Answer from the drawing. Dimensions are ordinates in mm from the lowest x, y and z of the part. A direction names the side the tool comes from. Give positions to 0.01 mm unless a question says otherwise; leave off trailing zeros. Loops run counter-clockwise (first coordinate to the right, second up) from the corner with the lowest first, then second, coordinate; pieces in that order, holes last. Notation, with made-up numbers: M 63.5,25 L 100.5,25 A25 cw 100.5,47 Z; hole C 28.25,82 d9. An arc over 180 degrees is marked long. Use a Markdown table: item, result.
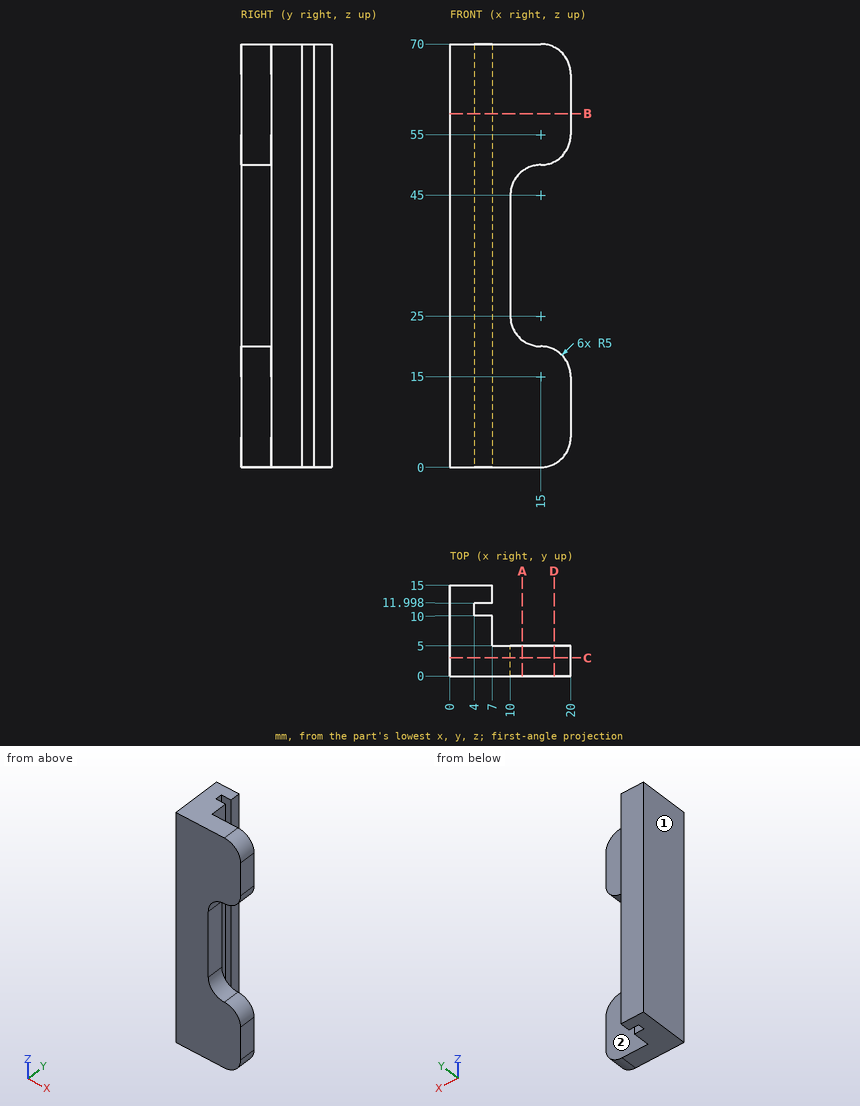
(1) Consider probe 1 along Y at (x, z) = (5, 40); probe 2 along X at (y, z) = (0.5, 34.5); probe 3 along X at (y, z) = (14.5, 66.5). Determine where each line is inside the solid, lowest interval first. Write a range as [from, to].
Entries:
| item | result |
|---|---|
| probe 1 | y = [0, 10], [12, 15] |
| probe 2 | x = [0, 10] |
| probe 3 | x = [0, 7] |
(2) A cutting plane is placed at B-B (z = 58.5). Write down the section's boundary in (x, y), and give its area (3 significant figures).
Entries:
| item | result |
|---|---|
| outline | M 0,0 L 20,0 L 20,5 L 7,5 L 7,10 L 4,10 L 4,12 L 7,12 L 7,15 L 0,15 Z |
| area | 164 mm² |
(3) Given P1, Ø4, axis at y = 8.5, z = 40.5, coming from the +X side; P2, Ø1.5, axis at y = 2, z = 30.5, coming from the +X side, each flat-ended and moving along its own axis, determine where each tip first touches the part or whether it passes through.
Entries:
| item | result |
|---|---|
| P1 | stops at x = 7 |
| P2 | stops at x = 10 |
(4) A cutting plane is placed at D-D (x = 17.25). Write down the section's boundary in (y, z) (3 decimals), and give its area (3 significant figures).
Entries:
| item | result |
|---|---|
| outline | M 0,0.535 L 5,0.535 L 5,19.465 L 0,19.465 Z; M 0,50.535 L 5,50.535 L 5,69.465 L 0,69.465 Z |
| area | 189 mm² |
(5) A cutting plane is placed at A-A (x = 12). Write down the section's boundary in (y, z).
Entries:
| item | result |
|---|---|
| outline | M 0,0 L 5,0 L 5,21 L 0,21 Z; M 0,49 L 5,49 L 5,70 L 0,70 Z |
(6) Which of the six approach directions +Z, -Z, +X, -X, +Y, -Y give full straight-line access (tool end or side, diameter ignored) to the marked faces 1 and 2?
Entries:
| item | result |
|---|---|
| face 1 | +Z, -Z, -X, +Y, -Y |
| face 2 | +Z, -Z, +X, +Y |
(7) A cutting plane is placed at C-C (y = 3). Write down the section's boundary in (x, z), and give its area (3 significant figures).
Entries:
| item | result |
|---|---|
| outline | M 0,0 L 15,0 A5 ccw 20,5 L 20,15 A5 ccw 15,20 A5 cw 10,25 L 10,45 A5 cw 15,50 A5 ccw 20,55 L 20,65 A5 ccw 15,70 L 0,70 Z |
| area | 1,090 mm² |
